Source: three-view drawing plus pictorial views. Frame: mm from the lowest corner of the part. Give positions to 0.01 mm unless a question says otherwise; leave off trailing zeros. Loops run counter-clockwise (first coordinate to the right, second up) from the corner with the lowest first, then second, coordinate; pieces in that order, holes last. Notation, with made-up numbers: (17.5, -29.5) -> (47.5, -29.5) arc R7 cw to (47.5, -23.5) -> close; hole circle Ø2 at (26.25, -7). An arc over 180 degrees is marked (long way). Answer as a JSON object with one key per item and string values. Group by question number.
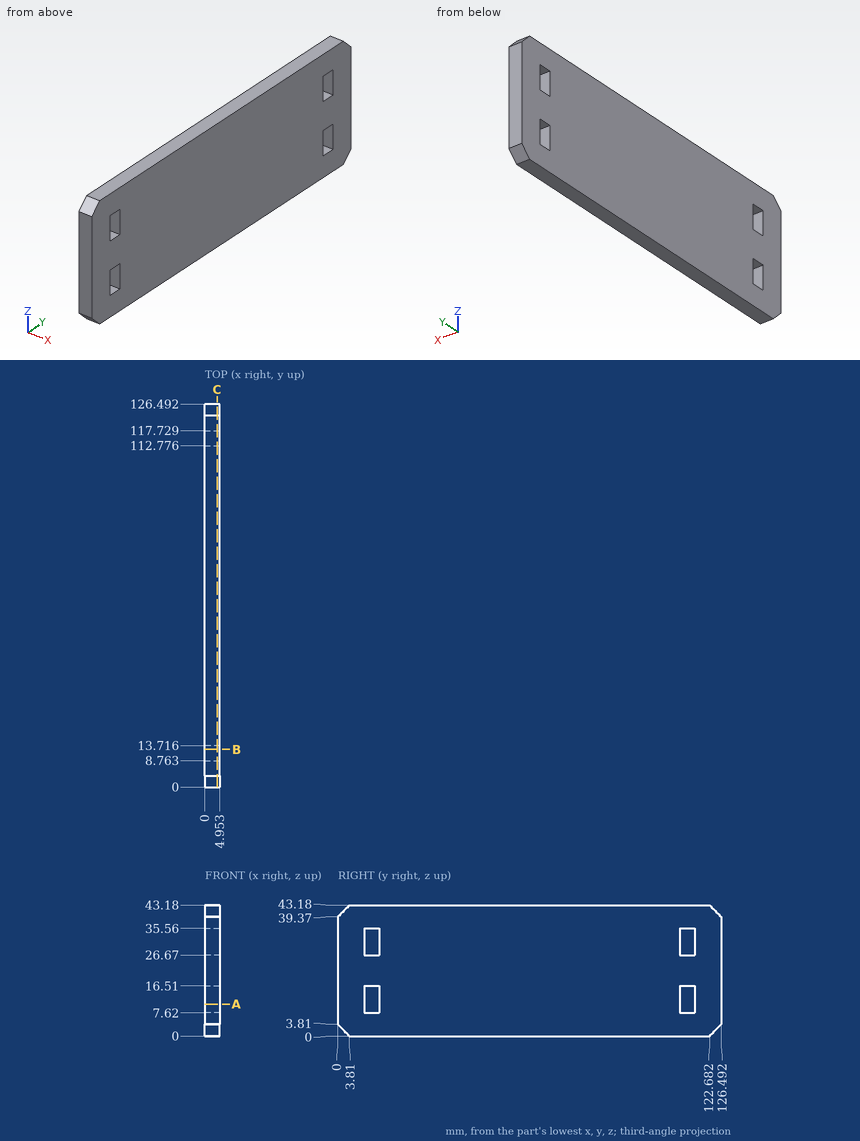
Q1. Section A-A on z = 10.5. Return the cut outline in (x, y).
Q2. Ray query, probe 1 along Y at (x, z) = (3.05, 32); probe 2 along Z at (x, y) = (2.7, 116.5). Return the intervals inside material, ascending.
Q3. Section B-B on y = 12.5. Return the cut outline in (x, z).
Q4. Section C-C on x = 4. Return the cut outline in (y, z), then the cut area to 3 significant figures.
Numbers:
{
 "1": {"outline": "(0, 0) -> (4.95, 0) -> (4.95, 8.76) -> (0, 8.76) -> close; (0, 13.72) -> (4.95, 13.72) -> (4.95, 112.78) -> (0, 112.78) -> close; (0, 117.73) -> (4.95, 117.73) -> (4.95, 126.49) -> (0, 126.49) -> close"},
 "2": {"probe 1": "y = 0 to 8.76, 13.72 to 112.78, 117.73 to 126.49", "probe 2": "z = 0 to 7.62, 16.51 to 26.67, 35.56 to 43.18"},
 "3": {"outline": "(0, 0) -> (4.95, 0) -> (4.95, 7.62) -> (0, 7.62) -> close; (0, 16.51) -> (4.95, 16.51) -> (4.95, 26.67) -> (0, 26.67) -> close; (0, 35.56) -> (4.95, 35.56) -> (4.95, 43.18) -> (0, 43.18) -> close"},
 "4": {"outline": "(0, 3.81) -> (3.81, 0) -> (122.68, 0) -> (126.49, 3.81) -> (126.49, 39.37) -> (122.68, 43.18) -> (3.81, 43.18) -> (0, 39.37) -> close; hole (8.76, 7.62) -> (13.72, 7.62) -> (13.72, 16.51) -> (8.76, 16.51) -> close; hole (8.76, 26.67) -> (13.72, 26.67) -> (13.72, 35.56) -> (8.76, 35.56) -> close; hole (112.78, 7.62) -> (117.73, 7.62) -> (117.73, 16.51) -> (112.78, 16.51) -> close; hole (112.78, 26.67) -> (117.73, 26.67) -> (117.73, 35.56) -> (112.78, 35.56) -> close", "area": "5,260 mm²"}
}
